```python
from build123d import *

# Parameters (mm, degrees)
F0_W     = 126.7150789499
F0_H     = 3.926018253
F0_H_2   = 6.0044974089
F0_W_2   = 48.0359867215
F0_W_3   = 17.5516083837
F0_H_3   = 43.8790284097
F0_W_4   = 38.5673493147
F1_DEPTH = 25.4


with BuildPart() as f1:
    # F0 (on Front) → F1 (new body)
    with BuildSketch(Plane.XZ):
        Polygon((0, 28.4861717373), (0, 0), (-13.9287291095, 0), (-13.9287291095, 28.4861717373), (-16.2381511182, 28.4861717373), (-16.2381511182, 0), (-39.3323749304, 0), (-39.3323749304, 28.4861717373), (-87.3683616519, 28.4861717373), (-87.3683616519, -53.2673746347), (126.7150789499, -53.2673746347), (126.7150789499, 28.4861717373), align=None)
        with Locations((63.357539475, 30.4491808638)):
            Rectangle(F0_W, F0_H)
        Polygon((126.7150789499, 32.4121899903), (126.7150789499, 28.4861717373), (205.0045132637, 28.4861717373), (205.0045132637, 82.2957158089), (126.7150789499, 82.2957158089), (126.7150789499, 76.2912184), (192.995518446, 76.2912184), (192.995518446, 32.4121899903), align=None)
        with Locations((63.357539475, 79.2934671044)):
            Rectangle(F0_W, F0_H_2)
        with Locations((-63.3503682911, 30.4491808638)):
            Rectangle(F0_W_2, F0_H)
        Polygon((0, 100.5401462317), (0, 82.2957158089), (126.7150789499, 82.2957158089), (126.7150789499, 116.2442192435), (-87.3683616519, 116.2442192435), (-87.3683616519, 82.2957158089), (-39.3323749304, 82.2957158089), (-39.3323749304, 100.5401462317), (-16.2381511182, 100.5401462317), (-16.2381511182, 82.2957158089), (-13.9287291095, 82.2957158089), (-13.9287291095, 100.5401462317), align=None)
        with Locations((-96.1441658437, 30.4491808638)):
            Rectangle(F0_W_3, F0_H)
        with Locations((-63.3503682911, 79.2934671044)):
            Rectangle(F0_W_2, F0_H_2)
        with Locations((-96.1441658437, 54.3517041951)):
            Rectangle(F0_W_3, F0_H_3)
        with Locations((-96.1441658437, 79.2934671044)):
            Rectangle(F0_W_3, F0_H_2)
        with Locations((-124.2036446929, 54.3517041951)):
            Rectangle(F0_W_4, F0_H_3)
    extrude(amount=F1_DEPTH)


solid = f1.part
```
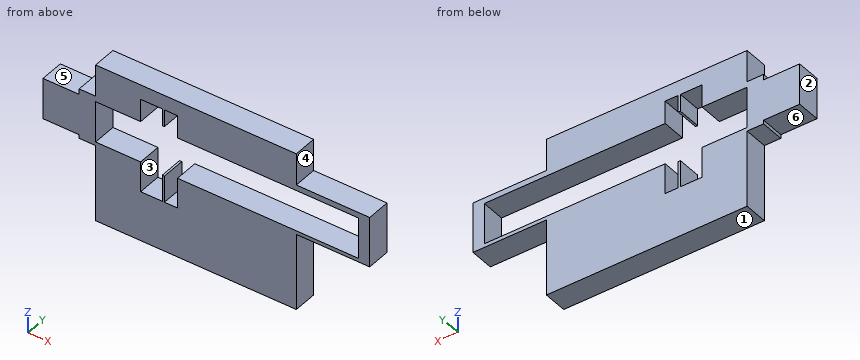
Can you work these out from the model? Positions are in its coordinate system, mm. Face numbers are marked on the shaded views. A direction names the side the tool comes from. Coordinates: 2 decimals unless noted, no trailing zeros. Loops run counter-clockwise (first coordinate to the right, second up) from the corner with the lowest first, then second, coordinate; pieces in that order, holes last. Notation, with made-up numbers: (-26.5, 87) - (30.5, 87) arc R6 cw to (30.5, 95) - close; hole circle Ø8 at (12, 30). An arc over 180 degrees is marked (long way). Answer as CSV lines item,"result". Start each with the question number.
1) Which directions (+Z, -Z, +X, -X, +Y, -Y) give clear straight access to the entire face, cutting with the end or side of a thin tool? Please do the marked faces 4, 5 and 6.
2) Suppose I cut it at C-C (z = 95). Please give me the cut outline in (x, y).
3) Suppose I cut it at B-B (x = -20). Please give me the cut outline in (y, z).
4) I need wall thicknesses on line 1 (X direction, y = -10.25, z = 18); line 2 (Z direction, x = 145, y = -22.75); line 3 (Z direction, x = 22.5, y = -2.5). Which ranges of each line are inside material? Lowest first, please. Write a range as from..to.
5) Thinking about a two-plate mould opening in X: for the marked faces 1, 2 and 3, which applies, pulls with the +X half, pulls with the -X half, needs draft (parallel to the pull), parting line crosses it, or undercut?
6) For pin 1 (14.5 mm diameter, centred on y = -8, z = 88, fed in from -X); pin 2 (12 mm diameter, centred on y = -10.5, z = 85.5, fed in from +X); pin 3 (3 mm diameter, centred on y = -7, z = -6.5, fed in from -X); pin 4 (8 mm diameter, centred on x = 151, y = -11, fed in from +Z), each with a flat end and sliding along its axis, tell me the tip position at first contact or that it passes through.
7) Suppose I cut it at D-D (x = -115.5). Please give me the cut outline in (y, z), plus the area to 3 significant figures.
8) Suppose I cut it at A-A (z = 64). Please give me the cut outline in (x, y).
Check result:
1,face 4,"+Z, +X, +Y, -Y"
1,face 5,"+Z, -X, +Y, -Y"
1,face 6,"-Z, -X, +Y, -Y"
2,outline,"(-87.37, -25.4) - (-39.33, -25.4) - (-39.33, 0) - (-87.37, 0) - close; (-16.24, -25.4) - (-13.93, -25.4) - (-13.93, 0) - (-16.24, 0) - close; (0, -25.4) - (126.72, -25.4) - (126.72, 0) - (0, 0) - close"
3,outline,"(-25.4, -53.27) - (0, -53.27) - (0, 0) - (-25.4, 0) - close; (-25.4, 100.54) - (0, 100.54) - (0, 116.24) - (-25.4, 116.24) - close"
4,line 1,"x = -87.37..-39.33, -16.24..-13.93, 0..126.72"
4,line 2,"z = 28.49..32.41, 76.29..82.3"
4,line 3,"z = -53.27..32.41, 76.29..116.24"
5,face 1,"needs draft"
5,face 2,"pulls with the -X half"
5,face 3,"undercut"
6,pin 1,"stops at x = -104.92"
6,pin 2,"stops at x = 205"
6,pin 3,"stops at x = -87.37"
6,pin 4,"stops at z = 82.3"
7,outline,"(-25.4, 32.41) - (0, 32.41) - (0, 76.29) - (-25.4, 76.29) - close"
7,area,"1,110 mm²"
8,outline,"(-143.49, -25.4) - (-87.37, -25.4) - (-87.37, 0) - (-143.49, 0) - close; (193, -25.4) - (205, -25.4) - (205, 0) - (193, 0) - close"
